from build123d import *

# Parameters (mm, degrees)
F0_R     = 8.318
F1_DEPTH = 6
F2_R     = 2.25
F3_DEPTH = 2
F5_DEPTH = 6
F6_COUNT = 30


with BuildPart() as f1:
    # F0 (on Top) → F1 (new body)
    with BuildSketch(Plane.XY):
        Circle(F0_R)
        Polygon((2.492998, 4.318), (4.985997, 0), (2.492998, -4.318), (-2.492998, -4.318), (-4.985997, 0), (-2.492998, 4.318), align=None, mode=Mode.SUBTRACT)
    extrude(amount=F1_DEPTH)

    # F2 (on face) → F3 (join)
    with BuildSketch(Plane.XY.offset(6)):
        Polygon((-4.985997, 0), (-2.492998, -4.318), (2.492998, -4.318), (4.985997, 0), (2.492998, 4.318), (-2.492998, 4.318), align=None)
        Circle(F2_R, mode=Mode.SUBTRACT)
    extrude(amount=-F3_DEPTH)


with BuildPart() as f5:
    # F4 (on face) → F5 (new body)
    with BuildSketch(Plane(origin=(0, 0, 0), x_dir=(1, 0, 0), z_dir=(0, 0, -1))):
        Polygon((-9.050051, 1), (-9.050051, -1), (-7.318, 0), align=None)
    extrude(amount=-F5_DEPTH)


with BuildPart() as f6_1:
    # F6: instance of F5
    add(f5.part.rotate(Axis((0, 0, 6), (0, 0, 1)), 1 * 360 / F6_COUNT))


with BuildPart() as f6_2:
    # F6: instance of F5
    add(f5.part.rotate(Axis((0, 0, 6), (0, 0, 1)), 2 * 360 / F6_COUNT))


with BuildPart() as f6_3:
    # F6: instance of F5
    add(f5.part.rotate(Axis((0, 0, 6), (0, 0, 1)), 3 * 360 / F6_COUNT))


with BuildPart() as f6_4:
    # F6: instance of F5
    add(f5.part.rotate(Axis((0, 0, 6), (0, 0, 1)), 4 * 360 / F6_COUNT))


with BuildPart() as f6_5:
    # F6: instance of F5
    add(f5.part.rotate(Axis((0, 0, 6), (0, 0, 1)), 5 * 360 / F6_COUNT))


with BuildPart() as f6_6:
    # F6: instance of F5
    add(f5.part.rotate(Axis((0, 0, 6), (0, 0, 1)), 6 * 360 / F6_COUNT))


with BuildPart() as f6_7:
    # F6: instance of F5
    add(f5.part.rotate(Axis((0, 0, 6), (0, 0, 1)), 7 * 360 / F6_COUNT))


with BuildPart() as f6_8:
    # F6: instance of F5
    add(f5.part.rotate(Axis((0, 0, 6), (0, 0, 1)), 8 * 360 / F6_COUNT))


with BuildPart() as f6_9:
    # F6: instance of F5
    add(f5.part.rotate(Axis((0, 0, 6), (0, 0, 1)), 9 * 360 / F6_COUNT))


with BuildPart() as f6_10:
    # F6: instance of F5
    add(f5.part.rotate(Axis((0, 0, 6), (0, 0, 1)), 10 * 360 / F6_COUNT))


with BuildPart() as f6_11:
    # F6: instance of F5
    add(f5.part.rotate(Axis((0, 0, 6), (0, 0, 1)), 11 * 360 / F6_COUNT))


with BuildPart() as f6_12:
    # F6: instance of F5
    add(f5.part.rotate(Axis((0, 0, 6), (0, 0, 1)), 12 * 360 / F6_COUNT))


with BuildPart() as f6_13:
    # F6: instance of F5
    add(f5.part.rotate(Axis((0, 0, 6), (0, 0, 1)), 13 * 360 / F6_COUNT))


with BuildPart() as f6_14:
    # F6: instance of F5
    add(f5.part.rotate(Axis((0, 0, 6), (0, 0, 1)), 14 * 360 / F6_COUNT))


with BuildPart() as f6_15:
    # F6: instance of F5
    add(f5.part.rotate(Axis((0, 0, 6), (0, 0, 1)), 15 * 360 / F6_COUNT))


with BuildPart() as f6_16:
    # F6: instance of F5
    add(f5.part.rotate(Axis((0, 0, 6), (0, 0, 1)), 16 * 360 / F6_COUNT))


with BuildPart() as f6_17:
    # F6: instance of F5
    add(f5.part.rotate(Axis((0, 0, 6), (0, 0, 1)), 17 * 360 / F6_COUNT))


with BuildPart() as f6_18:
    # F6: instance of F5
    add(f5.part.rotate(Axis((0, 0, 6), (0, 0, 1)), 18 * 360 / F6_COUNT))


with BuildPart() as f6_19:
    # F6: instance of F5
    add(f5.part.rotate(Axis((0, 0, 6), (0, 0, 1)), 19 * 360 / F6_COUNT))


with BuildPart() as f6_20:
    # F6: instance of F5
    add(f5.part.rotate(Axis((0, 0, 6), (0, 0, 1)), 20 * 360 / F6_COUNT))


with BuildPart() as f6_21:
    # F6: instance of F5
    add(f5.part.rotate(Axis((0, 0, 6), (0, 0, 1)), 21 * 360 / F6_COUNT))


with BuildPart() as f6_22:
    # F6: instance of F5
    add(f5.part.rotate(Axis((0, 0, 6), (0, 0, 1)), 22 * 360 / F6_COUNT))


with BuildPart() as f6_23:
    # F6: instance of F5
    add(f5.part.rotate(Axis((0, 0, 6), (0, 0, 1)), 23 * 360 / F6_COUNT))


with BuildPart() as f6_24:
    # F6: instance of F5
    add(f5.part.rotate(Axis((0, 0, 6), (0, 0, 1)), 24 * 360 / F6_COUNT))


with BuildPart() as f6_25:
    # F6: instance of F5
    add(f5.part.rotate(Axis((0, 0, 6), (0, 0, 1)), 25 * 360 / F6_COUNT))


with BuildPart() as f6_26:
    # F6: instance of F5
    add(f5.part.rotate(Axis((0, 0, 6), (0, 0, 1)), 26 * 360 / F6_COUNT))


with BuildPart() as f6_27:
    # F6: instance of F5
    add(f5.part.rotate(Axis((0, 0, 6), (0, 0, 1)), 27 * 360 / F6_COUNT))


with BuildPart() as f6_28:
    # F6: instance of F5
    add(f5.part.rotate(Axis((0, 0, 6), (0, 0, 1)), 28 * 360 / F6_COUNT))


with BuildPart() as f6_29:
    # F6: instance of F5
    add(f5.part.rotate(Axis((0, 0, 6), (0, 0, 1)), 29 * 360 / F6_COUNT))


with BuildPart() as f1_1:
    add(f1.part)

    # F7: cut F5, F6_1, F6_2, F6_3, F6_4, F6_5, F6_6, F6_7, F6_8, F6_9, F6_10, F6_11, F6_12, F6_13, F6_14, F6_15, F6_16, F6_17, F6_18, F6_19, F6_20, F6_21, F6_22, F6_23, F6_24, F6_25, F6_26, F6_27, F6_28, F6_29
    add(f5.part, mode=Mode.SUBTRACT)
    add(f6_1.part, mode=Mode.SUBTRACT)
    add(f6_2.part, mode=Mode.SUBTRACT)
    add(f6_3.part, mode=Mode.SUBTRACT)
    add(f6_4.part, mode=Mode.SUBTRACT)
    add(f6_5.part, mode=Mode.SUBTRACT)
    add(f6_6.part, mode=Mode.SUBTRACT)
    add(f6_7.part, mode=Mode.SUBTRACT)
    add(f6_8.part, mode=Mode.SUBTRACT)
    add(f6_9.part, mode=Mode.SUBTRACT)
    add(f6_10.part, mode=Mode.SUBTRACT)
    add(f6_11.part, mode=Mode.SUBTRACT)
    add(f6_12.part, mode=Mode.SUBTRACT)
    add(f6_13.part, mode=Mode.SUBTRACT)
    add(f6_14.part, mode=Mode.SUBTRACT)
    add(f6_15.part, mode=Mode.SUBTRACT)
    add(f6_16.part, mode=Mode.SUBTRACT)
    add(f6_17.part, mode=Mode.SUBTRACT)
    add(f6_18.part, mode=Mode.SUBTRACT)
    add(f6_19.part, mode=Mode.SUBTRACT)
    add(f6_20.part, mode=Mode.SUBTRACT)
    add(f6_21.part, mode=Mode.SUBTRACT)
    add(f6_22.part, mode=Mode.SUBTRACT)
    add(f6_23.part, mode=Mode.SUBTRACT)
    add(f6_24.part, mode=Mode.SUBTRACT)
    add(f6_25.part, mode=Mode.SUBTRACT)
    add(f6_26.part, mode=Mode.SUBTRACT)
    add(f6_27.part, mode=Mode.SUBTRACT)
    add(f6_28.part, mode=Mode.SUBTRACT)
    add(f6_29.part, mode=Mode.SUBTRACT)


solid = f1_1.part
The model under review builds one solid part; all positions refer to its coordinate system, in mm. A direction names the side the tool comes from. Round coordinates to 2 decimals unless told otherwise and drop trailing zeros. Order: outer loops, then holes, each group sorted by start corner. A loop starts at its lowest first (then second) coordinate and runs counter-clockwise, first axis right, second up. Notation, with made-up numbers: (-23.75, -28.75) - (-12.75, -28.75) arc R10 ccw to (-12.75, -11.75) - close; hole circle Ø7 at (48, 56). An arc over 180 degrees is marked (long way). Use one line per item in the form item = value.
Q1. Tool access review of faces 5 (the flat face through (3.72, 2.19, 1.97)), 6 (the flat face through (-7.69, 1.35, 2.96)), 7 (the flat face through (-6.49, -4.36, 2.96)), 8 (the flat face through (7.704, 1.344, 2.958)), 9 (the flat face through (-1.1, -7.74, 2.96)): name each direction out of +Z, -Z, +X, -X, +Y, -Y from which nothing blocks a thin tool from reaching the whole face with its end or side.
Response values:
face_5 = -Z
face_6 = +Z, -Z, -X
face_7 = +Z, -Z
face_8 = +Z, -Z, +X
face_9 = +Z, -Z, -Y
Q2. Mouldability with a two-part tool opening along X and no side actions: class faces 1 (the flat face through (5.4, -5.6, 3)), 2 (the flat face through (7.013, 3.428, 2.958)), 3 (the flat face through (-7.82, 0.29, 2.96)), 4 (the flat face through (-0.538, -7.788, 2.958)) as pulls with the +X half, pulls with the -X half, needs draft (parallel to the pull), parting line crosses it, or undercut.
Response values:
face_1 = undercut
face_2 = pulls with the +X half
face_3 = pulls with the -X half
face_4 = undercut
Q3. Add section B-B on y = 3.5. Give the boundary of the cut face in (x, z), then the cut area to 3 significant figures.
Response values:
outline = (-7.07, 0) - (-2.97, 0) - (-2.97, 4) - (2.97, 4) - (2.97, 0) - (7.07, 0) - (7.07, 6) - (-7.07, 6) - close
area = 61.1 mm^2
Q4. To check wall thickness, follow line 1 (Y direction, x = 0, z = 5.5); line 2 (Y direction, x = 6.25, z = 3.3); line 3 (Y direction, x = -0.5, z = 2.1). State the ranges of each line that lie inside material, in increasing order.
Response values:
line_1 = -8.32 to -2.25, 2.25 to 8.32
line_2 = -5.49 to -5.04, -4.34 to 4.34, 5.04 to 5.49
line_3 = -7.87 to -4.32, 4.32 to 7.87
Q5. Clearance check with flat-ended pins moving along their axes: P1, Ø2, axis at x = -5.5, z = 3.5, coming from the -Y side; P2, Ø2, axis at y = -5, z = 2, coming from the +X side; P3, Ø0.6, axis at y = 7, z = 2.5, coming from the -X side. State where each tip first meets the part, or that it passes through.
Response values:
P1 = -6.9
P2 = 7.29
P3 = -4.93
Q6. Add section A-A on x = 0. Give the boundary of the cut face in (y, z), then the cut area to 3 significant figures.
Response values:
outline = (-8.32, 0) - (-4.32, 0) - (-4.32, 4) - (-2.25, 4) - (-2.25, 6) - (-8.32, 6) - close; (2.25, 4) - (4.32, 4) - (4.32, 0) - (8.32, 0) - (8.32, 6) - (2.25, 6) - close
area = 56.3 mm^2
